```python
from build123d import *

# Parameters (mm, degrees)
SKETCH_1_W          = 37.5
SKETCH_1_H          = 22.5
EXTRUDE_2_DEPTH     = 4
SKETCH_2_W          = 15
SKETCH_2_H          = 10
EXTRUDE_3_DEPTH     = 18.5
EXTRUDE_4_DEPTH     = 15
EXTRUDE_5_DEPTH     = 8.66025404
SKETCH_5_R          = 1.7
CUT_EXTRUDE_1_DEPTH = 10
FILLET_1_R          = 15
FILLET_3_R          = 5
SKETCH_9_R          = 1.8
CUT_EXTRUDE_2_DEPTH = 4
FILLET_5_R          = 10
RIB_10_REACH        = 84.489
SKETCH_16_WALL_W    = 186.275176358
SKETCH_16_WALL_H    = 4
RIB_START           = -4
RIB_11_DEPTH        = 4


# Read off the part's stored shape, not the designer's step: the rib step
with BuildPart() as part:
    # Sketch 1 → Extrude 2 (new body)
    with BuildSketch(Plane(origin=(0, 0, 0), x_dir=(1, 0, 0), z_dir=(0, 1, 0))):
        with Locations((18.75, 11.25)):
            Rectangle(SKETCH_1_W, SKETCH_1_H)
    extrude(amount=EXTRUDE_2_DEPTH)

    # Sketch 2 → Extrude 3 (add)
    with BuildSketch(Plane(origin=(0, 4, 0), x_dir=(1, 0, 0), z_dir=(0, 1, 0))):
        with Locations((18.75, 11.25)):
            Rectangle(SKETCH_2_W, SKETCH_2_H)
    extrude(amount=EXTRUDE_3_DEPTH)

    # Sketch 3 → Extrude 4 (add)
    with BuildSketch(Plane(origin=(26.25, 0, 0), x_dir=(0, 0, -1), z_dir=(1, 0, 0))):
        Polygon((6.25, 22.5), (-17.75, 64.069219382), (-10.25, 68.399346401), (16.25, 22.5), align=None)
    extrude(amount=-EXTRUDE_4_DEPTH)

    # Sketch 4 → Extrude 5 (add)
    with BuildSketch(Plane(origin=(0, 8.331329387, -14.430285793), x_dir=(1, 0, 0), z_dir=(0, -0.5000000000000041, 0.8660254037844363))):
        with BuildLine():
            Line((26.25, 64.360571585), (11.25, 64.360571585))
            ThreePointArc((11.25, 64.360571585), (18.75, 71.860571585), (26.25, 64.360571585))
        make_face()
    extrude(amount=-EXTRUDE_5_DEPTH)

    # Sketch 5 → Cut-Extrude 1 (cut)
    with BuildSketch(Plane(origin=(0, 8.331329387, -14.430285793), x_dir=(1, 0, 0), z_dir=(0, -0.5000000000000041, 0.8660254037844363))):
        with Locations(Location((18.75, 64.360571585, 0), (0, 0, 270))):
            Circle(SKETCH_5_R)
        with Locations(Location((18.75, 27.360571585, 0), (0, 0, 270))):
            Circle(SKETCH_5_R)
    extrude(amount=-CUT_EXTRUDE_1_DEPTH, mode=Mode.SUBTRACT)

    # Fillet 1
    fillet_1_edges = [part.edges().sort_by_distance(p)[0] for p in [
        (18.75, 22.5, -6.25),
    ]]
    fillet(fillet_1_edges, radius=FILLET_1_R)

    # Fillet 3
    fillet_3_edges = [part.edges().sort_by_distance(p)[0] for p in [
        (0, 2, -22.5),
        (37.5, 2, -22.5),
        (37.5, 2, 0),
        (0, 2, 0),
    ]]
    fillet(fillet_3_edges, radius=FILLET_3_R)

    # Sketch 9 → Cut-Extrude 2 (cut)
    with BuildSketch(Plane(origin=(0, 4, 0), x_dir=(1, 0, 0), z_dir=(0, 1, 0))):
        with Locations(Location((5, 17.5, 0), (0, 0, 270))):
            Circle(SKETCH_9_R)
        with Locations(Location((32.5, 17.5, 0), (0, 0, 90))):
            Circle(SKETCH_9_R)
        with Locations(Location((32.5, 5, 0), (0, 0, 270))):
            Circle(SKETCH_9_R)
        with Locations(Location((5, 5, 0), (0, 0, 90))):
            Circle(SKETCH_9_R)
    extrude(amount=-CUT_EXTRUDE_2_DEPTH, mode=Mode.SUBTRACT)

    # Fillet 5
    fillet_5_edges = [part.edges().sort_by_distance(p)[0] for p in [
        (18.75, 22.5, -16.25),
    ]]
    fillet(fillet_5_edges, radius=FILLET_5_R)

    # Sketch 16 wall → Rib 10 (add, up to next)
    with BuildSketch(Plane(origin=(26.25, 13.079426042, -19.236382193), x_dir=(0, 0.941051653324, 0.33826289447), z_dir=(0, -0.33826289447, 0.941051653324)), mode=Mode.PRIVATE) as rib_10_sk1:
        with Locations((0, 2)):
            Rectangle(SKETCH_16_WALL_W, SKETCH_16_WALL_H)
    rib_10_tool1 = extrude(rib_10_sk1.sketch, amount=RIB_10_REACH, mode=Mode.PRIVATE) - part.part
    add(rib_10_tool1.solids().sort_by_distance((26.25, 13.079426042, -19.236382193))[0])

    # Rib 11 outline → Rib 11 (add)
    with BuildSketch(Plane.ZY.offset(-11.25).offset(RIB_START)):
        with BuildLine():
            Line((-15.98478303, 22.108301633), (-22.5, 4))
            Line((-22.5, 4), (-16.25, 4))
            Line((-16.25, 4), (-16.25, 19.820508076))
            ThreePointArc((-16.25, 19.820508076), (-16.183474475, 20.972065652), (-15.98478303, 22.108301633))
        make_face()
    extrude(amount=RIB_11_DEPTH)


solid = part.part
```
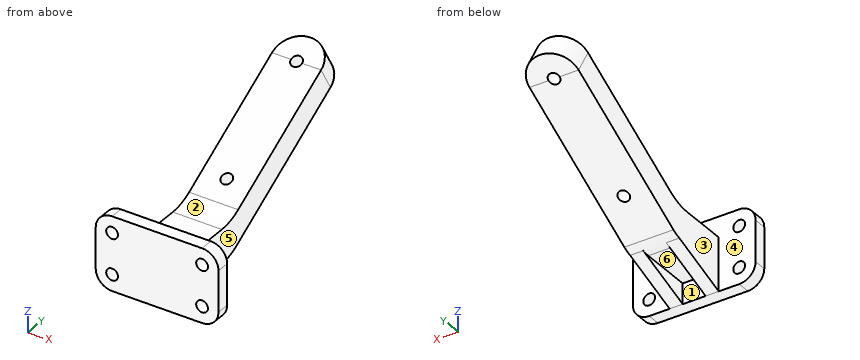
Here's how the part is built. I have some questions about the finished solid (model axes, mm). Face numbers are marked on the shaded views. A direction names the side the tool comes from. Coordinates: 2 decimals unless noted, no trailing zeros. Order: outer loops, then holes, each group sorted by start corner. A loop starts at its lowest first (then second) coordinate and runs counter-clockwise, first axis right, second up. Notation, with made-up numbers: (8, -1) -> (58, -1) arc R11 cw to (58, 7) -> close; hole circle Ø4 at (0, 5.25). An arc over 180 degrees is marked (long way). Return JSON: item names as keys, results as strings.
1) If we section it at D-D on z = 1: List the corners of the cut face in (x, y) for me.
Conclusion:
{"outline": "(11.25, 35.06) -> (26.25, 35.06) -> (26.25, 52.38) -> (11.25, 52.38) -> close"}
2) If we section it at A-A on z = -13: List the corners of the cut face in (x, y) for me, plus the area to 3 significant figures.
Conclusion:
{"outline": "(0, 0) -> (37.5, 0) -> (37.5, 4) -> (26.25, 4) -> (26.25, 28.13) -> (11.25, 28.13) -> (11.25, 4) -> (0, 4) -> close", "area": "512 mm²"}
3) If I drill on probe 1 along X at (y, z) = (1.55, -17.5); probe 2 along X at (y, z) = (2, -17); probe 3 along Y at (x, z) = (33.5, -11), over which ranges is the centre line in solid material (lowest first)?
Conclusion:
{"probe 1": "x = 0 to 3.2, 6.8 to 30.7, 34.3 to 37.5", "probe 2": "x = 0 to 3.27, 6.73 to 30.77, 34.23 to 37.5", "probe 3": "y = 0 to 4"}
4) If we section it at B-B on y = 16.5: List the corners of the cut face in (x, z) for me, plus the area to 3 significant figures.
Conclusion:
{"outline": "(11.25, -18) -> (15.25, -18) -> (15.25, -16.25) -> (22.25, -16.25) -> (22.25, -18.01) -> (26.25, -18.01) -> (26.25, -6.25) -> (11.25, -6.25) -> close", "area": "164 mm²"}
5) On a 3-axis mill with a long thin cutter (end or side, diameter ignored), from which of +Z, -Z, +X, -X, +Y, -Y can I reach the whole of each face in a straight line? I mean the marked faces 1, 2 and 3. Say none if no direction works.
Conclusion:
{"face 1": "-Z, +Y", "face 2": "+Z, +X, -X", "face 3": "+Z, -Z, -X, +Y"}
6) If we section it at C-C on x = 23.5: List the corners of the cut face in (y, z) for me, plus the area to 3 significant figures.
Conclusion:
{"outline": "(0, -22.5) -> (4, -22.5) -> (22.16, -15.97) arc R10 ccw to (24.82, -14.91) -> (73.43, 13.15) -> (69.1, 20.65) -> (25.98, -4.24) arc R15 cw to (18.48, -6.25) -> (4, -6.25) -> (4, 0) -> (0, 0) -> close", "area": "818 mm²"}
7) Thinking about a two-plate mould opening in X: for the marked faces 4, 5 and 6, which applies, +X half, -X half, draft (parallel to the pull), parting line (faces both ways), or undercut?
Conclusion:
{"face 4": "draft", "face 5": "+X half", "face 6": "undercut"}
8) I'm going to push flat-ended pins straight in: P1, Ø4, axis at x = 32.5, z = -5, coming from the -Y side; P2, Ø1.2, axis at x = 17.5, y = 1.5, coming from the +Z side; P3, Ø11.5, axis at x = 15, y = 12.5, coming from the +Z side; P4, Ø10, axis at x = 23, z = 7.5, coming from the -Y side. Where does each tip first touch, or does it pass through?
Conclusion:
{"P1": "stops at y = 0", "P2": "stops at z = 0", "P3": "stops at z = -6.25", "P4": "stops at y = 37.66"}
